Input: part model. Units: mm. Frame: model coordinates. Give positions to 0.01 mm unless a question says otherwise; leave off trailing zeros. Loops run counter-clockwise (first coordinate to the right, second up) from the corner with the lowest first, then second, coordinate; pieces in that order, holes last. Notation, with made-up numbers: M 69.5,-3.5 L 99.5,-3.5 A25 ccw 99.5,8.5 Z; hole C -24.5,-17 d3. An arc over 180 degrees is marked long. Return JSON: item names as keys, results as strings. Group by question number.
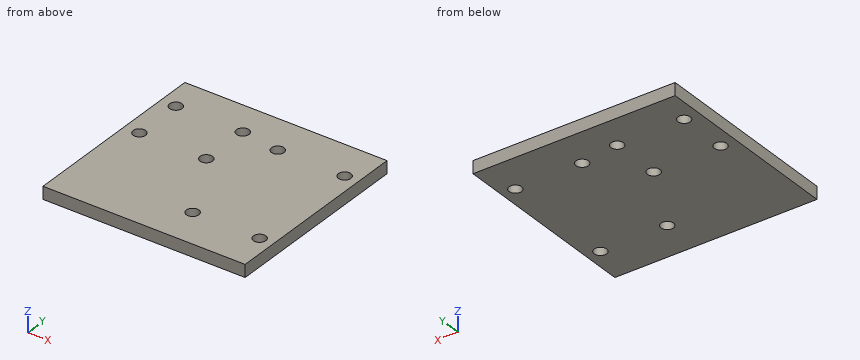
```python
from build123d import *

# Parameters (mm, degrees)
SKETCH1_W          = 72.5
SKETCH1_H          = 70
SKETCH1_R          = 2.25
BASE_FLANGE1_DEPTH = 4.5


# Sheet-metal steps are written as plain solids
with BuildPart() as part:
    # Sketch1 → Base-Flange1 (new body)
    with BuildSketch(Plane.XY):
        with Locations((-3.976149958, 1.616858374)):
            Rectangle(SKETCH1_W, SKETCH1_H)
        with Locations(Location((-34.726149958, 24.616858374, 0), (0, 0, 180))):
            Circle(SKETCH1_R, mode=Mode.SUBTRACT)
        with Locations(Location((-10.726149958, 24.616858374, 0), (0, 0, 180))):
            Circle(SKETCH1_R, mode=Mode.SUBTRACT)
        with Locations(Location((-10.726149958, 6.616858374, 0), (0, 0, 180))):
            Circle(SKETCH1_R, mode=Mode.SUBTRACT)
        with Locations(Location((-34.726149958, 6.616858374, 0), (0, 0, 180))):
            Circle(SKETCH1_R, mode=Mode.SUBTRACT)
        with Locations(Location((3.273850042, -19.383141626, 0), (0, 0, 180))):
            Circle(SKETCH1_R, mode=Mode.SUBTRACT)
        with Locations(Location((3.273850042, 22.616858374, 0), (0, 0, 180))):
            Circle(SKETCH1_R, mode=Mode.SUBTRACT)
        with Locations(Location((27.273850042, -19.383141626, 0), (0, 0, 180))):
            Circle(SKETCH1_R, mode=Mode.SUBTRACT)
        with Locations(Location((27.273850042, 22.616858374, 0), (0, 0, 180))):
            Circle(SKETCH1_R, mode=Mode.SUBTRACT)
    extrude(amount=-BASE_FLANGE1_DEPTH)


solid = part.part
```
Item 1: Material intervals for line 1 (Y direction, x = -10, z = -2.15); line 2 (X direction, y = -19.5, z = -4.1); line 3 (X direction, y = 25.5, z = -0.9), sorted ascending. Write a range as from..to.
Item 2: Section C-C, the plane z = -2.4. Give the number of separate pieces and of enclosed holes in the cut face, then the cut area to 3 significant figures.
Item 3: Section B-B, the plane x = -35. Return loops of the section in (y, z).
Item 4: First-contact query: pin 1 Ø5 at (x, y) = (-10.73, 24.62) entering from -Z. Flat tip, straight axial feed; report the tip coordinate or a pass-through.
Item 5: Section A-A, the plane y = 7.5. Return loops of the section in (x, z), then the cut area to 3 significant figures.
Answer below:
{
 "1": {"line 1": "-33.38..4.49, 8.75..22.49, 26.75..36.62", "line 2": "-40.23..1.03, 5.52..25.03, 29.52..32.27", "line 3": "-40.23..-36.8, -32.66..-12.8, -8.66..32.27"},
 "2": {"separate pieces": "1", "enclosed holes": "8", "area": "4,950 mm^2"},
 "3": {"outline": "M -33.38,-4.5 L 4.38,-4.5 L 4.38,0 L -33.38,0 Z; M 8.85,-4.5 L 22.38,-4.5 L 22.38,0 L 8.85,0 Z; M 26.85,-4.5 L 36.62,-4.5 L 36.62,0 L 26.85,0 Z"},
 "4": {"pin 1": "z = -4.5"},
 "5": {"outline": "M -40.23,-4.5 L -36.8,-4.5 L -36.8,0 L -40.23,0 Z; M -32.66,-4.5 L -12.8,-4.5 L -12.8,0 L -32.66,0 Z; M -8.66,-4.5 L 32.27,-4.5 L 32.27,0 L -8.66,0 Z", "area": "289 mm^2"}
}
